Can you work these out from the model? Positions are in its coordinate system, mm. Face numbers are marked on the shaded views. A direction names the side the tool comes from. Give positions to 0.01 mm unless a question says otherwise; leave off trailing zeros. Write each loop counter-clockwise with the first axis right and the second up, starting at its lowest first coordinate (ties: lowest second). Pieces come first, ordered by that corner, then holes.
1. I'm going to push flat-ended pins straight in: pin 1 (1.3 mm diameter, centred on y = -35, z = -12, fed in from +X); pin 2 (1.5 mm diameter, centred on y = 11.5, z = 3.5, fed in from +X); pin 3 (2.5 mm diameter, centred on x = -47, z = 4, fed in from +Y). Where does each tip first touch, or does it pass through?
2. Suppose I cut it at A-A (y = 12.5). Please give me the cut outline in (x, z).
3. If I drill on probe 1 along Y at (x, z) = (-14, -14.5); probe 2 along X at (y, z) = (21, -10.5); probe 3 along Z at (x, y) = (-41.5, 10), over which ranges is the centre line in solid material (lowest first)?
4. On a 3-axis mill with a long thin cutter (end or side, diameter ignored), from which of +Z, -Z, +X, -X, +Y, -Y can I reach the whole of each face in a straight line? I mean the marked faces 1 and 2. Say none if no direction works.
5. Suppose I cut it at C-C (z = -26.5). Please give me the cut outline in (x, y), and give its area (3 significant figures).
6. Thinking about a two-plate mould opening in Z: for the marked faces 3, 4 and 5, which applies, pulls with the +Z half, pulls with the -Z half, needs draft (parallel to the pull), parting line crosses it, or undercut?
7. Suppose I cut it at D-D (y = 45.5). Please give me the cut outline in (x, z).
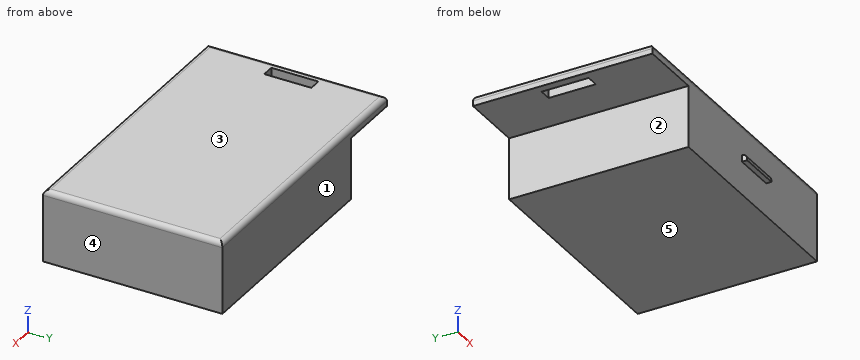
```python
from build123d import *

# Parameters (mm, degrees)
F0_W     = 142.1354152262
F0_H     = 88.716968894
F1_DEPTH = 5.08
F2_W     = 6.1184130609
F2_H     = 23.2970286161
F3_DEPTH = 25.4
F4_W     = 110.9326332808
F4_H     = 88.716968894
F5_DEPTH = 30.48
F6_W     = 20.9437925369
F6_H     = 3.2945293933
F7_DEPTH = 2.54
F8_R     = 2.54
F9_R     = 2.53999


# Not quite as in the source:
# - a fillet or chamfer is up to 0.001 mm smaller than in the source, because OpenCascade refuses the exact size


with BuildPart() as f1:
    # F0 (on Top) → F1 (new body)
    with BuildSketch(Plane.XY):
        with Locations((16.7079698294, 10.4718953371)):
            Rectangle(F0_W, F0_H)
    extrude(amount=F1_DEPTH)

    # F2 (on face) → F3 (cut)
    with BuildSketch(Plane.XY.offset(5.08)):
        with Locations((-47.1599567682, 11.648514308)):
            Rectangle(F2_W, F2_H)
    extrude(amount=-F3_DEPTH, mode=Mode.SUBTRACT)

    # F4 (on face) → F5 (join)
    with BuildSketch(Plane(origin=(0, 0, 0), x_dir=(1, 0, 0), z_dir=(0, 0, -1))):
        with Locations((32.3093608022, -10.4718953371)):
            Rectangle(F4_W, F4_H)
    extrude(amount=F5_DEPTH)

    # F6 (on face) → F7 (join)
    with BuildSketch(Plane.XZ.offset(33.8865891099)):
        with Locations((33.4383537993, -12.4721480533)):
            Rectangle(F6_W, F6_H)
    extrude(amount=F7_DEPTH)

    # F8
    f8_edges = [f1.edges().sort_by_distance(p)[0] for p in [
        (16.70797, -33.886589, 5.08),
        (-54.359738, 10.471895, 5.08),
        (16.70797, 54.83038, 5.08),
        (87.775677, 10.471895, 5.08),
    ]]
    fillet(f8_edges, radius=F8_R)

    # F9 (radius 2.54 in the source; OpenCascade refuses exactly that, so slightly less here)
    f9_edges = [f1.edges().sort_by_distance(p)[0] for p in [
        (33.438354, -36.426589, -10.824883),
    ]]
    fillet(f9_edges, radius=F9_R)


solid = f1.part
```
Checks:
1. pin 1: stops at x = 43.91
1. pin 2: stops at x = 87.77
1. pin 3: stops at y = 54.82
2. outline: (-54.36, 0) - (-50.22, 0) - (-50.22, 5.08) - (-51.82, 5.08) arc R2.54 ccw to (-54.36, 2.54) - close; (-44.1, 0) - (-23.16, 0) - (-23.16, -30.48) - (87.78, -30.48) - (87.78, 2.54) arc R2.54 ccw to (85.24, 5.08) - (-44.1, 5.08) - close
3. probe 1: y = -33.89 to 54.83
3. probe 2: x = -23.16 to 87.78
3. probe 3: z = 0 to 5.08
4. face 1: +Z, -Z, +X, -X, +Y
4. face 2: -Z, -X, +Y, -Y
5. outline: (-23.16, -33.89) - (87.78, -33.89) - (87.78, 54.83) - (-23.16, 54.83) - close
5. area: 9,840 mm2
6. face 3: pulls with the +Z half
6. face 4: needs draft
6. face 5: pulls with the -Z half
7. outline: (-54.36, 0) - (-23.16, 0) - (-23.16, -30.48) - (87.78, -30.48) - (87.78, 2.54) arc R2.54 ccw to (85.24, 5.08) - (-51.82, 5.08) arc R2.54 ccw to (-54.36, 2.54) - close
